For this review, take the finished solid that the model builds, in its own axes (mm). A direction names the side the tool comes from. Coordinates: 2 decimals unless noted, no trailing zeros. Order: outer loops, then holes, each group sorted by start corner. A loop starts at its lowest first (then second) coordinate and runs counter-clockwise, first axis right, second up. Notation, with made-up numbers: (11, -38) - (21, -38) arc R17 ccw to (21, -25) - close; hole circle Ø3 at (48, 57). An arc over 180 degrees is marked (long way). One line per item, written item: value. Start each with the question number.
(1) Consider section B-B on x = 23.5. Write out the cut boundary in (y, z).
(2) For faces 1 (the flat face through (19, 33, 3)), 2 (the flat face through (26, 8, 2)), 3 (the flat face through (57, 5, 2)), 4 (the flat face through (22, 0, 2)), list the 3-axis set-ups (+Z, -Z, +X, -X, +Y, -Y) from which the entire face can be reached by the end or side of a thin tool; tool diameter is ignored.
(3) Mouldability with a two-part tool opening along X and no side actions: class faces 5 (the flat face through (57, 25, 2)), 6 (the flat face through (21, 34, 3)), 7 (the cylindrical face through (45.93, -8.5, 2.54)) as released by +X, released by -X, zero draft, split by the parting line, or undercut.
(4) Consider section C-C on y = 14. Write out the cut boundary in (x, z), then the cut area to 4 significant figures.
(5) Consider section A-A on y = 37.5. Write out the cut boundary in (x, z).
(6) To check wall thickness, follow line 1 along Y through (x, z) = (57, 1.25); line 2 along Y through (x, z) = (22.5, 4.6); line 3 along Y through (x, z) = (55.5, 3.4). State the ranges of each line that lie inside material, in increasing order.
(7) Clearance check with flat-ended pins moving along their axes: pin 1 (2.5 mm diameter, centred on x = 19.5, z = 2, fed in from +Y); pin 2 (2.5 mm diameter, centred on x = 28.5, z = 3, fed in from +Y); pin 3 (3 mm diameter, centred on x = 27.5, z = 3.5, fed in from -Y). State where each tip first meets the part, or that it passes through.
(8) Consider section D-D on z = 4.3. Count the separate pieces of the cut face and the enclosed holes in it, then the cut area to 3 significant figures.
```python
from build123d import *

# Parameters (mm, degrees)
SKETCH1_R           = 6.35
SKETCH1_R_2         = 1.2
SKETCH1_W           = 10
SKETCH1_H           = 17.5
BOSS_EXTRUDE1_DEPTH = 5
SKETCH2_W           = 3
SKETCH2_H           = 2
CUT_EXTRUDE1_DEPTH  = 72.869673716
FILLET1_R           = 5


with BuildPart() as part:
    # Sketch1 → Boss-Extrude1 (new body)
    with BuildSketch(Plane.XY):
        Polygon((0, 40), (15, 40), (15, 35), (26, 35), (37, 35), (37, 40), (59.5, 40), (59.5, 25), (54.5, 25), (54.5, 5), (59.5, 5), (59.5, -10), (44.5, -10), (44.5, 0), (0, 0), align=None)
        with Locations((12, 24.5)):
            Circle(SKETCH1_R, mode=Mode.SUBTRACT)
        with Locations((44, 24.5)):
            Circle(SKETCH1_R, mode=Mode.SUBTRACT)
        with Locations((7.5, 37.5)):
            Circle(SKETCH1_R_2, mode=Mode.SUBTRACT)
        with Locations((44.5, 37.5)):
            Circle(SKETCH1_R_2, mode=Mode.SUBTRACT)
        with Locations((57, 32.5)):
            Circle(SKETCH1_R_2, mode=Mode.SUBTRACT)
        with Locations((57, -2.5)):
            Circle(SKETCH1_R_2, mode=Mode.SUBTRACT)
        with Locations((26, 16.75)):
            Rectangle(SKETCH1_W, SKETCH1_H, mode=Mode.SUBTRACT)
    extrude(amount=BOSS_EXTRUDE1_DEPTH)

    # Sketch2 → Cut-Extrude1 (cut, through all)
    with BuildSketch(Plane.XY.offset(5)):
        with Locations((19.5, 34)):
            Rectangle(SKETCH2_W, SKETCH2_H)
        with Locations((32.5, 34)):
            Rectangle(SKETCH2_W, SKETCH2_H)
    extrude(amount=-CUT_EXTRUDE1_DEPTH, mode=Mode.SUBTRACT)

    # Fillet1
    fillet1_edges = [part.edges().sort_by_distance(p)[0] for p in [
        (44.5, -10, 2.5),
        (44.5, 0, 2.5),
        (0, 0, 2.5),
    ]]
    fillet(fillet1_edges, radius=FILLET1_R - 0.0001)  # a hair under: the kernel refuses the full size


solid = part.part
```
Geometry check:
1. outline: (0, 0) - (8, 0) - (8, 5) - (0, 5) - close; (25.5, 0) - (35, 0) - (35, 5) - (25.5, 5) - close
2. face 1: +Z, -Z, +Y
2. face 2: +Z, -Z
2. face 3: +Z, -Z, +X
2. face 4: +Z, -Z, -X, -Y
3. face 5: zero draft
3. face 6: undercut
3. face 7: released by -X
4. outline: (0, 0) - (21, 0) - (21, 5) - (0, 5) - close; (31, 0) - (54.5, 0) - (54.5, 5) - (31, 5) - close
4. area: 222.5 mm^2
5. outline: (0, 0) - (6.3, 0) - (6.3, 5) - (0, 5) - close; (8.7, 0) - (15, 0) - (15, 5) - (8.7, 5) - close; (37, 0) - (43.3, 0) - (43.3, 5) - (37, 5) - close; (45.7, 0) - (59.5, 0) - (59.5, 5) - (45.7, 5) - close
6. line 1: y = -10 to -3.7, -1.3 to 5, 25 to 31.3, 33.7 to 40
6. line 2: y = 0 to 8, 25.5 to 35
6. line 3: y = -10 to 5, 25 to 40
7. pin 1: stops at y = 33
7. pin 2: stops at y = 35
7. pin 3: stops at y = 0
8. separate pieces: 1
8. enclosed holes: 7
8. area: 1,860 mm^2
